```python
from build123d import *

# Parameters (mm, degrees)
F0_R     = 3.25
F1_DEPTH = 3


with BuildPart() as f1:
    # F0 (on Front) → F1 (new body)
    with BuildSketch(Plane.XZ):
        with BuildLine():
            ThreePointArc((350, 345), (348.535534, 348.535534), (345, 350))
            Line((345, 350), (-345, 350))
            ThreePointArc((-345, 350), (-348.535534, 348.535534), (-350, 345))
            Line((-350, 345), (-350, -345))
            ThreePointArc((-350, -345), (-348.535534, -348.535534), (-345, -350))
            Line((-345, -350), (345, -350))
            ThreePointArc((345, -350), (348.535534, -348.535534), (350, -345))
            Line((350, -345), (350, 345))
        make_face()
        with Locations((-312.5, -337.5)):
            Circle(F0_R, mode=Mode.SUBTRACT)
        with Locations((-337.5, -312.5)):
            Circle(F0_R, mode=Mode.SUBTRACT)
        with Locations((-187.5, -337.5)):
            Circle(F0_R, mode=Mode.SUBTRACT)
        with Locations((-337.5, -187.5)):
            Circle(F0_R, mode=Mode.SUBTRACT)
        with Locations((-62.5, -337.5)):
            Circle(F0_R, mode=Mode.SUBTRACT)
        with BuildLine():
            Line((-44.644661, -75), (44.644661, -75))
            ThreePointArc((44.644661, -75), (46.558078, -75.380602), (48.180195, -76.464466))
            Line((48.180195, -76.464466), (288.180195, -316.464466))
            ThreePointArc((288.180195, -316.464466), (289.264059, -321.913417), (284.644661, -325))
            Line((284.644661, -325), (-284.644661, -325))
            ThreePointArc((-284.644661, -325), (-289.264059, -321.913417), (-288.180195, -316.464466))
            Line((-288.180195, -316.464466), (-48.180195, -76.464466))
            ThreePointArc((-48.180195, -76.464466), (-46.558078, -75.380602), (-44.644661, -75))
        make_face(mode=Mode.SUBTRACT)
        with Locations((-337.5, -62.5)):
            Circle(F0_R, mode=Mode.SUBTRACT)
        with Locations((62.5, -337.5)):
            Circle(F0_R, mode=Mode.SUBTRACT)
        with Locations((187.5, -337.5)):
            Circle(F0_R, mode=Mode.SUBTRACT)
        with Locations((312.5, -337.5)):
            Circle(F0_R, mode=Mode.SUBTRACT)
        with Locations((337.5, -312.5)):
            Circle(F0_R, mode=Mode.SUBTRACT)
        with Locations((337.5, -187.5)):
            Circle(F0_R, mode=Mode.SUBTRACT)
        with BuildLine():
            Line((75, -44.644661), (75, 44.644661))
            ThreePointArc((75, 44.644661), (75.380602, 46.558078), (76.464466, 48.180195))
            Line((76.464466, 48.180195), (316.464466, 288.180195))
            ThreePointArc((316.464466, 288.180195), (321.913417, 289.264059), (325, 284.644661))
            Line((325, 284.644661), (325, -284.644661))
            ThreePointArc((325, -284.644661), (321.913417, -289.264059), (316.464466, -288.180195))
            Line((316.464466, -288.180195), (76.464466, -48.180195))
            ThreePointArc((76.464466, -48.180195), (75.380602, -46.558078), (75, -44.644661))
        make_face(mode=Mode.SUBTRACT)
        with Locations((337.5, -62.5)):
            Circle(F0_R, mode=Mode.SUBTRACT)
        with Locations((-337.5, 62.5)):
            Circle(F0_R, mode=Mode.SUBTRACT)
        with BuildLine():
            Line((-75, 44.644661), (-75, -44.644661))
            ThreePointArc((-75, -44.644661), (-75.380602, -46.558078), (-76.464466, -48.180195))
            Line((-76.464466, -48.180195), (-316.464466, -288.180195))
            ThreePointArc((-316.464466, -288.180195), (-321.913417, -289.264059), (-325, -284.644661))
            Line((-325, -284.644661), (-325, 284.644661))
            ThreePointArc((-325, 284.644661), (-321.913417, 289.264059), (-316.464466, 288.180195))
            Line((-316.464466, 288.180195), (-76.464466, 48.180195))
            ThreePointArc((-76.464466, 48.180195), (-75.380602, 46.558078), (-75, 44.644661))
        make_face(mode=Mode.SUBTRACT)
        with Locations((-337.5, 187.5)):
            Circle(F0_R, mode=Mode.SUBTRACT)
        with Locations((-337.5, 312.5)):
            Circle(F0_R, mode=Mode.SUBTRACT)
        with Locations((-312.5, 337.5)):
            Circle(F0_R, mode=Mode.SUBTRACT)
        with Locations((-187.5, 337.5)):
            Circle(F0_R, mode=Mode.SUBTRACT)
        with Locations((-62.5, 337.5)):
            Circle(F0_R, mode=Mode.SUBTRACT)
        with Locations((337.5, 62.5)):
            Circle(F0_R, mode=Mode.SUBTRACT)
        with BuildLine():
            Line((44.644661, 75), (-44.644661, 75))
            ThreePointArc((-44.644661, 75), (-46.558078, 75.380602), (-48.180195, 76.464466))
            Line((-48.180195, 76.464466), (-288.180195, 316.464466))
            ThreePointArc((-288.180195, 316.464466), (-289.264059, 321.913417), (-284.644661, 325))
            Line((-284.644661, 325), (284.644661, 325))
            ThreePointArc((284.644661, 325), (289.264059, 321.913417), (288.180195, 316.464466))
            Line((288.180195, 316.464466), (48.180195, 76.464466))
            ThreePointArc((48.180195, 76.464466), (46.558078, 75.380602), (44.644661, 75))
        make_face(mode=Mode.SUBTRACT)
        with Locations((62.5, 337.5)):
            Circle(F0_R, mode=Mode.SUBTRACT)
        with Locations((337.5, 187.5)):
            Circle(F0_R, mode=Mode.SUBTRACT)
        with Locations((187.5, 337.5)):
            Circle(F0_R, mode=Mode.SUBTRACT)
        with Locations((337.5, 312.5)):
            Circle(F0_R, mode=Mode.SUBTRACT)
        with Locations((312.5, 337.5)):
            Circle(F0_R, mode=Mode.SUBTRACT)
    extrude(amount=F1_DEPTH)


solid = f1.part
```
The model under review builds one solid part; all positions refer to its coordinate system, in mm. A direction names the side the tool comes from. Round coordinates to 2 decimals unless told otherwise and drop trailing zeros. Loops run counter-clockwise (first coordinate to the right, second up) from the corner with the lowest first, then second, coordinate; pieces in that order, holes last. Notation, with made-up numbers: (18, 47.5) - (31, 47.5) arc R9 ccw to (31, 54.5) - close; hole circle Ø9 at (28, 37.5). An arc over 180 degrees is marked (long way). Write each question's results on one line, items separated by ' | '. Start each with the question number.
Q1. Take a section at B-B on x = -201. Give the boundary of the cut face in (y, z).
Q2. Take a section at C-C on z = -87.5. Give the boundary of the cut face in (x, y).
Q3. Take a section at D-D on y = -1.55. Give the number of separate pieces and of enclosed holes in the cut face, plus the area to 3 significant figures.
Q4. Take a section at A-A on z = 25. Give the boundary of the cut face in (x, y).
Q5. Insertion check: P1, Ø5, axis at x = 187.5, z = 337.5, coming from the +Y side. The pin has a flat end and moves straight along its axis. Give the tip position at first contact, or say it passes through.
Q6. Draft analysis for pull direction Z (two halves, no side actions). For faces 1 (the flat face through (-2, -3, -24)), 2 (the flat face through (-198.144, -1.479, 169.86)), state which applies: pulls with the +Z half, pulls with the -Z half, needs draft (parallel to the pull), parting line crosses it, or undercut.
Q7. Tool access review of faces 3 (the flat face through (-194.784, -1.479, -166.5)), 4 (the flat face through (-2, 0, -24)): name each direction out of +Z, -Z, +X, -X, +Y, -Y from which nothing blocks a thin tool from reaching the whole face with its end or side.
Q8. Wall thickness on line 1 along X through (y, z) = (-1.25, -4); line 2 along Z through (x, y) = (-130.5, -0.4): over which ranges is each line inside the solid? List them lowest first. Write a range as [from, to].
Data:
1) outline: (-3, -350) - (0, -350) - (0, -325) - (-3, -325) - close; (-3, -229.28) - (0, -229.28) - (0, -172.72) - (-3, -172.72) - close; (-3, 172.72) - (0, 172.72) - (0, 229.28) - (-3, 229.28) - close; (-3, 325) - (0, 325) - (0, 350) - (-3, 350) - close
2) outline: (-350, -3) - (-325, -3) - (-325, 0) - (-350, 0) - close; (-115.78, -3) - (-59.22, -3) - (-59.22, 0) - (-115.78, 0) - close; (59.22, -3) - (115.78, -3) - (115.78, 0) - (59.22, 0) - close; (325, -3) - (350, -3) - (350, 0) - (325, 0) - close
3) separate pieces: 1 | enclosed holes: 28 | area: 146,000 mm²
4) outline: (-350, -3) - (-325, -3) - (-325, 0) - (-350, 0) - close; (-75, -3) - (75, -3) - (75, 0) - (-75, 0) - close; (325, -3) - (350, -3) - (350, 0) - (325, 0) - close
5) P1: passes through
6) face 1: needs draft | face 2: undercut
7) face 3: +Y, -Y | face 4: +Z, -Z, +X, -X, +Y
8) line 1: x = [-350, -325], [-75, 75], [325, 350] | line 2: z = [-350, -325], [-158.78, -102.22], [102.22, 158.78], [325, 350]
